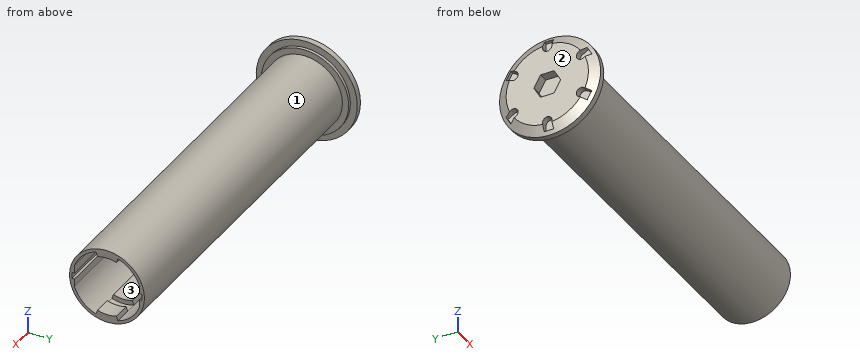
from build123d import *

# Parameters (mm, degrees)
F3_DEPTH        = 112
F4_R            = 12
F5_DEPTH        = 112.5
F7_DEPTH        = 3
F9_DEPTH        = 2
F9_COPIES_COUNT = 6
F11_START       = 57.5
F10_R           = 11
F11_DEPTH       = 3.5
F12_DEPTH       = 100


# Not quite as in the source:
# - a pattern or mirror of a feature is missing from the dataset's text; its kind, count and spacing are read off the source's solid


with BuildPart() as f1:
    # F0 (on Front) → F1 (revolve)
    with BuildSketch(Plane.XZ):
        Polygon((-50, 13.2), (-50, 0), (-46, 0), (-46, 11), (66.5, 11), (66.5, 12), (-45.6, 12), (-45.6, 14), (-46.6, 14), (-46.6, 16.2), (-48.4, 16.2), align=None)
    revolve(axis=Axis((3.169978948, 0, 0), (1, 0, 0)))

    # F2 (on face) → F3 (cut)
    with BuildSketch(Plane.YZ.offset(66.5)):
        with BuildLine():
            ThreePointArc((-10.9544511501, -1), (-11, 0), (-10.9544511501, 1))
            Line((-10.9544511501, 1), (-11.25, 1))
            Line((-11.25, 1), (-11.25, -1))
            Line((-11.25, -1), (-10.9544511501, -1))
        make_face()
        with BuildLine():
            Line((11.25, 1), (10.9544511501, 1))
            ThreePointArc((10.9544511501, 1), (10.9886068874, 0.5005184057), (11, 0))
            ThreePointArc((11, 0), (10.9886068874, -0.5005184057), (10.9544511501, -1))
            Line((10.9544511501, -1), (11.25, -1))
            Line((11.25, -1), (11.25, 1))
        make_face()
    extrude(amount=-F3_DEPTH, mode=Mode.SUBTRACT)

    # F4 (on face) → F5 (join, through all)
    with BuildSketch(Plane.YZ.offset(66.5)):
        Circle(F4_R)
        with BuildLine():
            ThreePointArc((-10.4544511501, 3.4211768662), (-7.8074781011, 7.7487602686), (-3.5, 10.4283268073))
            ThreePointArc((-3.5, 10.4283268073), (0, 11), (3.5, 10.4283268073))
            ThreePointArc((3.5, 10.4283268073), (7.8074781011, 7.7487602686), (10.4544511501, 3.4211768662))
            ThreePointArc((10.4544511501, 3.4211768662), (10.7726876303, 2.2246800266), (10.9544511501, 1))
            Line((10.9544511501, 1), (11.25, 1))
            Line((11.25, 1), (11.25, -1))
            Line((11.25, -1), (10.9544511501, -1))
            ThreePointArc((10.9544511501, -1), (10.7726876303, -2.2246800266), (10.4544511501, -3.4211768662))
            ThreePointArc((10.4544511501, -3.4211768662), (7.8074781011, -7.7487602686), (3.5, -10.4283268073))
            ThreePointArc((3.5, -10.4283268073), (0, -11), (-3.5, -10.4283268073))
            ThreePointArc((-3.5, -10.4283268073), (-7.8074781011, -7.7487602686), (-10.4544511501, -3.4211768662))
            ThreePointArc((-10.4544511501, -3.4211768662), (-10.7726876303, -2.2246800266), (-10.9544511501, -1))
            Line((-10.9544511501, -1), (-11.25, -1))
            Line((-11.25, -1), (-11.25, 1))
            Line((-11.25, 1), (-10.9544511501, 1))
            ThreePointArc((-10.9544511501, 1), (-10.7726876303, 2.2246800266), (-10.4544511501, 3.4211768662))
        make_face(mode=Mode.SUBTRACT)
        with BuildLine():
            ThreePointArc((3.5, 10.4283268073), (0, 11), (-3.5, 10.4283268073))
            Line((-3.5, 10.4283268073), (-3.0227272727, 9.0062822427))
            ThreePointArc((-3.0227272727, 9.0062822427), (0, 9.5), (3.0227272727, 9.0062822427))
            Line((3.0227272727, 9.0062822427), (3.5, 10.4283268073))
        make_face()
        with BuildLine():
            Line((-3.0227272727, -9.0062822427), (-3.5, -10.4283268073))
            ThreePointArc((-3.5, -10.4283268073), (0, -11), (3.5, -10.4283268073))
            Line((3.5, -10.4283268073), (3.0227272727, -9.0062822427))
            ThreePointArc((3.0227272727, -9.0062822427), (0, -9.5), (-3.0227272727, -9.0062822427))
        make_face()
    extrude(amount=-F5_DEPTH)

    # F6 (on face) → F7 (cut)
    with BuildSketch(Plane(origin=(-50, 0, 0), x_dir=(0, -1, 0), z_dir=(-1, 0, 0))):
        Polygon((-4.3301270189, 0), (-2.1650635095, -3.75), (2.1650635095, -3.75), (4.3301270189, 0), (2.1650635095, 3.75), (-2.1650635095, 3.75), align=None)
    extrude(amount=-F7_DEPTH, mode=Mode.SUBTRACT)

    # F8 (on face) → F9 (cut)
    with BuildSketch(Plane(origin=(-50, 0, 0), x_dir=(0, -1, 0), z_dir=(-1, 0, 0))):
        with BuildLine():
            Line((1.5, 15), (-1.5, 15))
            Line((-1.5, 15), (-1.5, 12.5))
            ThreePointArc((-1.5, 12.5), (0, 11), (1.5, 12.5))
            Line((1.5, 12.5), (1.5, 15))
        make_face()
    f9 = extrude(amount=-F9_DEPTH, mode=Mode.SUBTRACT)

    # F9_copies: F9 ×6 about axis
    f9_copies_axis = Axis((0, 0, 0), (1, 0, 0))
    for i in range(1, F9_COPIES_COUNT):
        add(f9.rotate(f9_copies_axis, i * 360 / F9_COPIES_COUNT), mode=Mode.SUBTRACT)

    # F10 (on Right) → F11 (cut)
    with BuildSketch(Plane.YZ.offset(F11_START)):
        Circle(F10_R)
    extrude(amount=F11_DEPTH, mode=Mode.SUBTRACT)

    # F2 (on face) → F12 (join)
    with BuildSketch(Plane.YZ.offset(66.5)):
        with BuildLine():
            Line((10.4544511501, 1), (10.9544511501, 1))
            ThreePointArc((10.9544511501, 1), (10.7726876303, 2.2246800266), (10.4544511501, 3.4211768662))
            Line((10.4544511501, 3.4211768662), (10.4544511501, 1))
        make_face()
        with BuildLine():
            ThreePointArc((10.4544511501, -3.4211768662), (10.7726876303, -2.2246800266), (10.9544511501, -1))
            Line((10.9544511501, -1), (10.4544511501, -1))
            Line((10.4544511501, -1), (10.4544511501, -3.4211768662))
        make_face()
        with BuildLine():
            ThreePointArc((-10.9544511501, -1), (-10.7726876303, -2.2246800266), (-10.4544511501, -3.4211768662))
            Line((-10.4544511501, -3.4211768662), (-10.4544511501, -1))
            Line((-10.4544511501, -1), (-10.9544511501, -1))
        make_face()
        with BuildLine():
            Line((-10.4544511501, 1), (-10.4544511501, 3.4211768662))
            ThreePointArc((-10.4544511501, 3.4211768662), (-10.7726876303, 2.2246800266), (-10.9544511501, 1))
            Line((-10.9544511501, 1), (-10.4544511501, 1))
        make_face()
    extrude(amount=-F12_DEPTH)


solid = f1.part
Check sheet for the modelled part. Datum: model origin and axes. Units: mm. Face numbers are marked on the shaded views. Give positions to 0.01 mm unless a question says otherwise; leave off trailing zeros. Write each loop counter-clockwise with the first axis right and the second up, starting at its lowest first coordinate (ties: lowest second). Pieces come first, ordered by that corner, then holes. Notation, with made-up numbers: (18.5, -13.75) -> (50.5, -13.75) arc R23 ccw to (50.5, 5.25) -> close; hole circle Ø3 at (68, 50). An arc over 180 degrees is marked (long way). One line per item, written item: value. Start each with the question number.
Item 1: Draft check along Z on the marked faces 1, 2 and 3. Enter one of: +Z half, -Z half, draft (parallel to the pull), parting line (faces both ways), or undercut.
Item 2: Section check A-A on x = 49. Record the cut outline in (y, z).
Item 3: Material ranges on probe 1 along Z at (x, y) = (51, 0.5); probe 2 along X at (y, z) = (8.5, -3); probe 3 along Y at (x, z) = (-13.5, -2.5), recorded low to high. Write a range as from..to.
Item 4: Gauge pin test, flat ends, axial feed: pin 1 (2.5 mm diameter, centred on x = 12.5, z = 2, fed in from -Y); pin 2 (4 mm diameter, centred on x = -11, y = 10, fed in from -Z); pin 3 (1 mm diameter, centred on x = -29, y = -11, fed in from +Z). Record the tip position at first contact, or that the pin passes through.
Results list:
1. face 1: parting line
1. face 2: draft
1. face 3: undercut
2. outline: circle Ø24 at (0, 0); hole (-11.25, -1) -> (-10.45, -1) -> (-10.45, -3.42) arc R11 ccw to (-3.5, -10.43) -> (-3.02, -9.01) arc R9.5 ccw to (3.02, -9.01) -> (3.5, -10.43) arc R11 ccw to (10.45, -3.42) -> (10.45, -1) -> (11.25, -1) -> (11.25, 1) -> (10.45, 1) -> (10.45, 3.42) arc R11 ccw to (3.5, 10.43) -> (3.02, 9.01) arc R9.5 ccw to (-3.02, 9.01) -> (-3.5, 10.43) arc R11 ccw to (-10.45, 3.42) -> (-10.45, 1) -> (-11.25, 1) -> close
3. probe 1: -11.99..-9.49, 9.49..11.99
3. probe 2: -50..-46
3. probe 3: -11.74..-10.45, 10.45..11.74
4. pin 1: y = -11.98
4. pin 2: z = -8.94
4. pin 3: z = 5.81
